The model under review builds one solid part; all positions refer to its coordinate system, in mm. Face numbers are marked on the shaded views. A direction names the side the tool comes from. Coordinates: 2 decimals unless noted, no trailing zeros. Order: outer loops, then holes, each group sorted by start corner. A loop starts at its lowest first (then second) coordinate and runs counter-clockwise, first axis right, second up.
from build123d import *

# Parameters (mm, degrees)
F0_W     = 70.4970285296
F0_H     = 70.4970285296
F1_DEPTH = 34.925
F2_T     = -6.35
F3_R     = 5.08
F4_SIZE  = 2.54


with BuildPart() as f1:
    # F0 (on Top) → F1 (new body, symmetric)
    with BuildSketch(Plane.XY):
        Rectangle(F0_W, F0_H)
    extrude(amount=F1_DEPTH, both=True)

    # F2
    f2_openings = [f1.faces().sort_by_distance(p)[0] for p in [
        (0, 0, 34.925),
    ]]
    offset(amount=F2_T, openings=f2_openings)

    # F3
    f3_edges = [f1.edges().sort_by_distance(p)[0] for p in [
        (0, 35.248514, -34.925),
        (0, -35.248514, -34.925),
        (35.248514, 0, -34.925),
        (-35.248514, 0, -34.925),
        (0, -28.898514, -28.575),
        (28.898514, 0, -28.575),
        (-28.898514, 0, -28.575),
        (0, 28.898514, -28.575),
        (35.248514, -35.248514, 0),
        (35.248514, 35.248514, 0),
        (-35.248514, 35.248514, 0),
        (-35.248514, -35.248514, 0),
        (-28.898514, 28.898514, 3.175),
        (28.898514, 28.898514, 3.175),
        (28.898514, -28.898514, 3.175),
        (-28.898514, -28.898514, 3.175),
    ]]
    fillet(f3_edges, radius=F3_R)

    # F4
    f4_edges = [f1.edges().sort_by_distance(p)[0] for p in [
        (-35.248514, 0, 34.925),
    ]]
    chamfer(f4_edges, length=F4_SIZE)


solid = f1.part
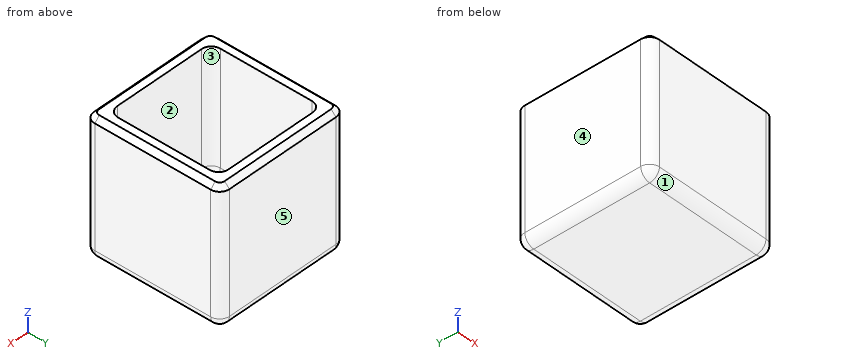
(1) The part is to be moulded in two halves that separate along Y. For the marked faces 3, 4 and 5, say which applies: +Y half, -Y half, draft (parallel to the pull), parting line (faces both ways), or undercut.
(2) Consider section A-A (z = 1.5). Give the boundary of the cut face in (x, y).
(3) Tool access review of the marked faces 1 and 2: name each direction out of +Z, -Z, +X, -X, +Y, -Y from which nothing blocks a thin tool from reaching the whole face with its end or side.
(4) Wall thickness on line 1 (X direction, y = -14, z = -21.5); line 2 (Z direction, x = -22, y = 19) (3 decimals): over which ranges is each line inside the solid? List them lowest first.
(5) Insertion check: pin 1 Ø10 at (x, y) = (14, -9.5) entering from +Z (3 decimals); pin 2 Ø6 at (x, y) = (-12.5, -26) entering from +Z (3 decimals). Each pin has a flat end and moves straight along its axis. Give the tip position at first contact, or say it passes through.
(6) Consider section B-B (y = -19.5). Give the boundary of the cut face in (x, z) (3 decimals).
Findings:
1. face 3: undercut
1. face 4: draft
1. face 5: +Y half
2. outline: (-35.25, -30.17) arc R5.08 ccw to (-30.17, -35.25) - (30.17, -35.25) arc R5.08 ccw to (35.25, -30.17) - (35.25, 30.17) arc R5.08 ccw to (30.17, 35.25) - (-30.17, 35.25) arc R5.08 ccw to (-35.25, 30.17) - close; hole (-28.9, -23.82) arc R5.08 ccw to (-23.82, -28.9) - (23.82, -28.9) arc R5.08 ccw to (28.9, -23.82) - (28.9, 23.82) arc R5.08 ccw to (23.82, 28.9) - (-23.82, 28.9) arc R5.08 ccw to (-28.9, 23.82) - close
3. face 1: -Z, +X, -X, -Y
3. face 2: +Z
4. line 1: x = -35.25 to -28.9, 28.9 to 35.25
4. line 2: z = -34.925 to -28.575
5. pin 1: stops at z = -28.575
5. pin 2: stops at z = 34.925
6. outline: (-35.249, -29.845) arc R5.08 ccw to (-30.169, -34.925) - (30.169, -34.925) arc R5.08 ccw to (35.249, -29.845) - (35.249, 32.385) - (32.709, 34.925) - (28.899, 34.925) - (28.899, -23.495) arc R5.08 cw to (23.819, -28.575) - (-23.819, -28.575) arc R5.08 cw to (-28.899, -23.495) - (-28.899, 34.925) - (-32.709, 34.925) - (-35.249, 32.385) - close
